Autodesk Inventor part; units mm, degrees
ref_plane "Work Plane1" through (0, 0, -26.75) normal (0, 0, -1) x (-1, 0, 0)
ref_plane "Work Plane2" through (18, 0, 0) normal (1, 0, 0) x (0, 1, 0)
ref_plane "Work Plane3" through (0, 0, 26.5) normal (0, 0, -1) x (-1, 0, 0)
sketch "Sketch1" plane through (0, 0, 0) normal (0, 0, 1) x (1, 0, 0)
  circle A0 centre (0, 0) radius 17.9
  dimension "d0" = 35.8
extrude "Extrusion1" add sketch "Sketch1" along normal mid plane 57
fillet "Fillet1" radius 2 1 edges at (-17.9, 0, 28.5)
shell "Shell1" thickness 0.62 removed faces 1 at (-5.8627, 4.3009, -28.5)
sketch "Sketch2" plane through (0, 0, 28.5) normal (0, 0, 1) x (1, 0, 0)
  circle A0 centre (0, 0) radius 15.9
  circle A1 centre (0, 0) radius 6.5
  dimension "d5" = 13
extrude "Extrusion2" add sketch "Sketch2" along normal blind 4.5 contours A1
fillet "Fillet2" radius 0.5 2 edges at (-6.5, 0, 28.5) (-6.5, 0, 33)
sketch "Sketch3" plane through (0, 0, 33) normal (0, 0, 1) x (1, 0, 0)
  circle A0 centre (0, 0) radius 6
  circle A1 centre (0, 0) radius 1.6
  dimension "d9" = 3.2
extrude "Extrusion3" add sketch "Sketch3" along normal blind 7.6 contours A1
fillet "Fillet3" radius 1.6 1 edges at (-1.6, 0, 40.6)
sketch "Sketch4" plane through (0, 0, 28.5) normal (0, 0, 1) x (1, 0, 0)
  circle A0 centre (0, 0) radius 15.9
  point P0 (12.5, 0)
  dimension "d13" = 12.5
hole "Hole1" at (12.5, 0, 28.5) direction (0, 0, -1) diameter 2.5 depth 8 tip angle 118
mirror "Mirror1" about plane through (0, 0, 0) normal (1, 0, 0) of "Hole1"
sketch "Sketch5" plane through (0, 0, 28.5) normal (0, 0, 1) x (1, 0, 0)
  circle A0 centre (12.5, 0) radius 1.25
  circle A1 centre (0, 0) radius 7
  arc A2 (13.523, 3.6235) -> (3.6235, 13.523) centre (0, 0) ccw
  arc A3 (9.6593, 2.5882) -> (2.5882, 9.6593) centre (0, 0) ccw
  line L0 (0, 0) -> (3.6235, 13.523) construction
  line L1 (0, 0) -> (13.523, 3.6235) construction
  line L2 (2.5882, 9.6593) -> (3.6235, 13.523)
  line L3 (9.6593, 2.5882) -> (13.523, 3.6235)
  line L4 (0, 0) -> (12.5, 0) construction
  line L5 (0.151, 0.5634) -> (0.151, 14.7153) construction
  dimension "d21" = 15
  dimension "d22" = 15
  dimension "d23" = 14
  dimension "d24" = 10
extrude "Extrusion4" cut sketch "Sketch5" against normal blind 10 contours L3 A3 L2 A2
pattern_circular "Circular Pattern1" count 4 over 360 about axis through (0, 0, 0) along (0, 0, 1) of "Extrusion4"
ref_plane "Work Plane1" through (0, 0, -26.75) normal (0, 0, -1) x (-1, 0, 0)
sketch "Sketch6" plane through (0, 0, -26.75) normal (0, 0, -1) x (-1, 0, 0)
  circle A0 centre (0, 0) radius 17.28
extrude "Extrusion5" add sketch "Sketch6" against normal blind 0.62
sketch "Sketch7" plane through (0, 0, -26.75) normal (0, 0, -1) x (-1, 0, 0)
  circle A0 centre (0, 0) radius 17.28
  circle A1 centre (0, 0) radius 12
  dimension "d33" = 24
extrude "Extrusion6" add sketch "Sketch7" along normal blind 0.62 contours A1
sketch "Sketch8" plane through (0, 0, -27.37) normal (0, 0, -1) x (-1, 0, 0)
  circle A0 centre (0, 0) radius 12
  circle A1 centre (0, 0) radius 5.375
  dimension "d36" = 10.75
extrude "Extrusion7" add sketch "Sketch8" along normal blind 3 contours A1
sketch "Sketch9" plane through (0, 0, -30.37) normal (0, 0, -1) x (-1, 0, 0)
  circle A0 centre (0, 0) radius 5.375
  circle A1 centre (0, 0) radius 3.45
  dimension "d39" = 6.9
extrude "Extrusion8" cut sketch "Sketch9" against normal blind 0.8 contours A1
sketch "Sketch10" plane through (0, 0, -29.57) normal (0, 0, -1) x (-1, 0, 0)
  circle A0 centre (0, 0) radius 3.45
  circle A1 centre (0, 0) radius 1.6
  dimension "d42" = 3.2
extrude "Extrusion9" add sketch "Sketch10" along normal blind 1 contours A1
sketch "Sketch11" plane through (0, 0, -27.37) normal (0, 0, -1) x (-1, 0, 0)
  circle A0 centre (0, 0) radius 5.375
  circle A1 centre (0, 0) radius 12
  arc A2 (9.3591, 3.15) -> (3.15, 9.3591) centre (0, 0) ccw
  arc A3 (5.6857, 3.15) -> (3.15, 5.6857) centre (0, 0) ccw
  line L0 (3.15, 9.3591) -> (3.15, 5.6857)
  line L1 (5.6857, 3.15) -> (9.3591, 3.15)
  dimension "d45" = 3.15
  dimension "d46" = 3.15
  dimension "d47" = 9.875
  dimension "d48" = 6.5
extrude "Extrusion10" cut sketch "Sketch11" against normal blind 1 contours L1 A3 L0 A2
pattern_circular "Circular Pattern2" count 4 over 360 about axis through (0, 0, 0) along (0, 0, 1) of "Extrusion10"
sketch "Sketch12" plane through (0, 0, -26.75) normal (0, 0, -1) x (-1, 0, 0)
  circle A0 centre (0, 0) radius 12
  circle A1 centre (0, 0) radius 17.28
  line L0 (-14.5, 1.9) -> (-14, 1.9)
  line L1 (-14, 1.9) -> (-14, -1.9)
  line L2 (-14, -1.9) -> (-14.5, -1.9)
  line L3 (-14.5, -1.9) -> (-14.5, 1.9)
  line L4 (0, 0) -> (-16.9017, 0) construction
  point P0 (-14, 0)
  dimension "d54" = 0.5
  dimension "d55" = 3.8
  dimension "d56" = 14
extrude "Extrusion11" add sketch "Sketch12" along normal blind 7.2 contours L0 L1 L2 L3
chamfer "Chamfer1" distance 1 angle 45 2 edges at (14.25, 1.9, -33.95) (14.25, -1.9, -33.95)
sketch "Sketch13" plane through (14.5, -1.9, -26.75) normal (1, 0, 0) x (0, 0, -1)
  line L0 (7.2, 1) -> (7.2, 2.8)
  line L1 (4.2, 1.9) -> (6.2, 3.8) construction
  line L2 (4.2, 1.9) -> (6.2, 0) construction
  dimension "d61" = 3
hole "Hole2" at (14.5, 0, -30.95) direction (-1, 0, 0) diameter 2 depth 1 tip angle 118
mirror "Mirror2" about plane through (0, 0, 0) normal (1, 0, 0) of "Extrusion11", "Chamfer1", "Hole2"
ref_plane "Work Plane2" through (18, 0, 0) normal (1, 0, 0) x (0, 1, 0)
sketch "Sketch14" plane through (18, 0, 0) normal (1, 0, 0) x (0, 1, 0)
  arc A0 (-6.7054, -11.85) -> (-6.7054, -17.75) centre (-6.7054, -14.8) ccw
  arc A1 (5.2946, -17.75) -> (5.2946, -11.85) centre (5.2946, -14.8) ccw
  line L0 (-6.7054, -11.85) -> (5.2946, -11.85)
  line L1 (-6.7054, -17.75) -> (5.2946, -17.75)
  line L2 (17.9, -28.5) -> (-17.9, -28.5)
  line L3 (0, -28.5) -> (0, 17.1564) construction
  dimension "d70" = 10.75
  dimension "d71" = 5.9
  dimension "d72" = 12
extrude "Extrusion12" cut sketch "Sketch14" against normal through all
ref_plane "Work Plane3" through (0, 0, 26.5) normal (0, 0, -1) x (-1, 0, 0)
sketch "Sketch15" plane through (0, 0, 26.5) normal (0, 0, -1) x (-1, 0, 0)
  circle A0 centre (0, 0) radius 17.9
  circle A1 centre (0, 0) radius 19.25
  dimension "d76" = 1.35
extrude "Flux Ring" add sketch "Sketch15" along normal blind 36.5
properties part number "RS-550" material "Steel, Mild"
Build history of the part. All positions in model axes, mm. A direction names the side the tool comes from. Give positions to 0.01 mm unless a question says otherwise; leave off trailing zeros. Loops run counter-clockwise (first coordinate to the right, second up) from the corner with the lowest first, then second, coordinate; pieces in that order, holes last. Notation, with made-up numbers: (21, 63.25) - (30, 63.25) arc R23 ccw to (30, 85.25) - close; hole circle Ø5 at (72.25, -29.5). An arc over 180 degrees is marked (long way). Use a Markdown table: item, result.
(1) Drop flat-ended pins along their axis: pin 1 Ø3 at (x, y) = (12, 6) entering from -Z; pin 2 Ø6 at (y, z) = (13.5, -22.5) entering from +X; pin 3 Ø0.5 at (x, z) = (7.5, -27) entering from -Y. Give the stop position or say it passes through.
Taken from the geometry:
| item | result |
|---|---|
| pin 1 | z = -27.37 |
| pin 2 | x = 14.5 |
| pin 3 | y = -16.37 |
(2) Which spindle directions (+Z, -Z, +X, -X, +Y, -Y) get a long thin tool onto all of the face, cutting with end or side? Do faces 1 (the face through (-14.25, 0.04, -29.95)), 2 (the face through (-13.74, 0.16, 28.19)), 3 (the face through (-13, -13, -10)), 4 (the face through (14.88, -9.655, -14.778)). Say none if no direction does.
Taken from the geometry:
| item | result |
|---|---|
| face 1 | -X |
| face 2 | +Z |
| face 3 | -Z |
| face 4 | +X, -X |
(3) Band-saw the part on A-A (z = -14.8). Give the cut face in (x, y), and give its area (3 significant figures).
Taken from the geometry:
| item | result |
|---|---|
| outline | (-15.89, 8.24) - (-15.19, 8.24) arc R17.28 cw to (15.19, 8.24) - (15.89, 8.24) arc R17.9 ccw to start; (-15.07, -9.66) arc R17.9 ccw to (15.07, -9.66) - (14.33, -9.66) arc R17.28 cw to (-14.33, -9.66) - close |
| area | 45.2 mm2 |
(4) Wall check: line 1 along Z through (x, y) = (14.2, 0); line 2 along Z through (x, y) = (6, 14.5); line 3 along Y through (x, z) = (0, 12). Give the ranges that are in metal, low to high.
Taken from the geometry:
| item | result |
|---|---|
| line 1 | -33.95 to -31.95, -29.95 to -26.13, 27.88 to 28.5 |
| line 2 | -26.75 to -26.13, 27.88 to 28.5 |
| line 3 | -19.25 to -17.28, 17.28 to 19.25 |
(5) Pull direction X, two halves, no side cores. Call faces 5 (the face through (14.25, -0.04, -29.95)), 6 (the face through (15.28, 11.71, 8.51)), 7 (the face through (0, 0, 27.88)): +X half, -X half, draft (parallel to the pull), parting line (faces both ways), or undercut.
Taken from the geometry:
| item | result |
|---|---|
| face 5 | draft |
| face 6 | parting line |
| face 7 | undercut |
(6) Band-saw the part on C-C (y = -8). Give the number of separate pieces and of enclosed holes in the cut face, and give its area (3 significant figures).
Taken from the geometry:
| item | result |
|---|---|
| separate pieces | 4 |
| enclosed holes | 0 |
| area | 217 mm2 |
(7) Band-saw the part on B-B (z = 25). Give the cut face in (x, y), and give its area (3 significant figures).
Taken from the geometry:
| item | result |
|---|---|
| outline | circle Ø38.5 at (0, 0); hole circle Ø34.56 at (0, 0) |
| area | 226 mm2 |
